Input: dimensioned drawing with shaded views. Units: mm. Origin: part minimum x, y, z. A direction names the side the tool comes from. Coordinates: 2 decimals unless noted, no trailing zeros. Loops run counter-clockwise (first coordinate to the right, second up) from the corner with the lowest first, then second, coordinate; pieces in that order, holes last. Notation, with made-up numbers: M 85.5,-13.5 L 133.5,-13.5 A36 cw 133.5,23.5 Z; hole C -10.5,44.5 d11. An arc over 180 degrees is marked long. Write item = value, one per line. Start each with the question number.
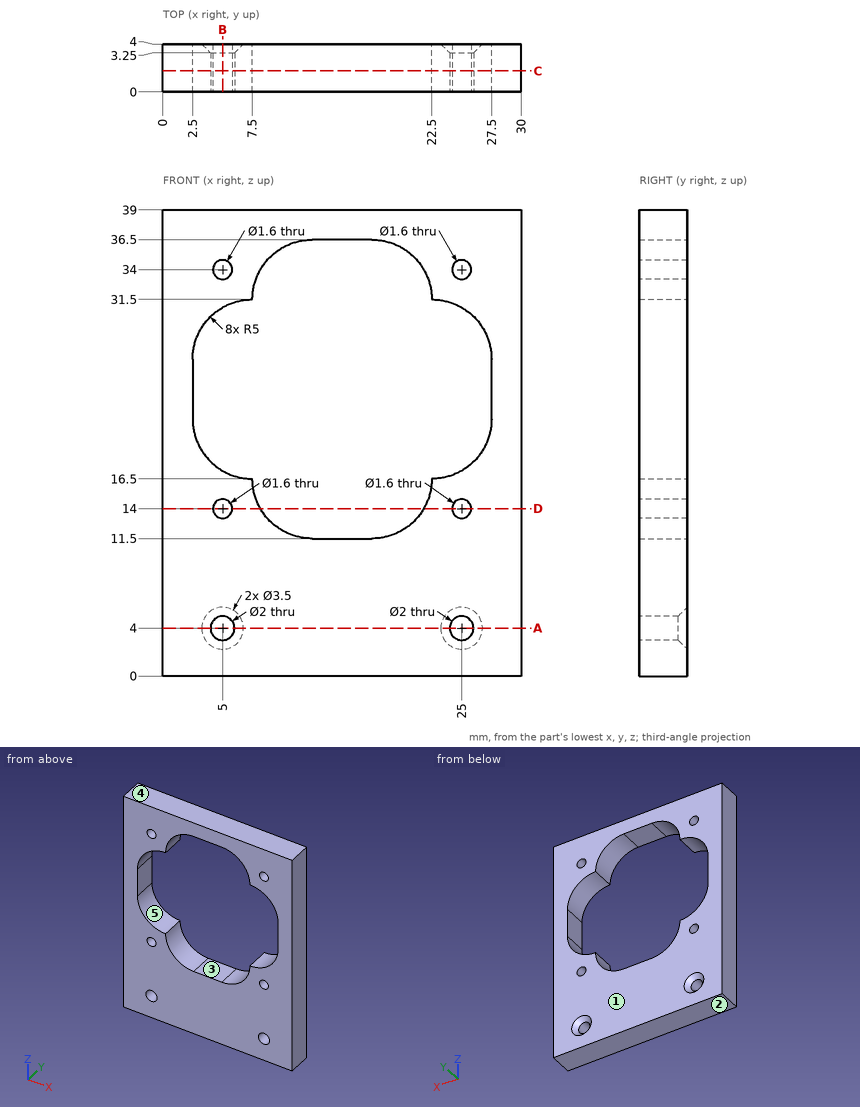
Item 1: Line query: line 1 (Z direction, x = 15.5, y = 1.6); line 2 (X direction, y = 2.85, z = 34); line 3 (Z direction, x = 25, y = 0.9). Output: solid intervals per line, ascending. Write a range as from..to.
Item 2: Pull-direction query (Z, two-part tool) for the marked faces 1, 2 and 3; classes: released by +Z, released by -Z, zero draft, split by the parting line, or undercut.
Item 3: Reachability of the marked faces 4 and 5 from +Z, -Z, +X, -X, +Y, -Y: full face, straight path, thin tool, end or side. Return the list, or none.
Item 4: Section query D-D (z = 14). Return the cut outline in (x, y).
Item 5: Section query C-C (y = 1.75). Count the separate pieces of the cut face and the enclosed holes in it, plus the area to 3 significant figures.
Item 6: Section query A-A (z = 4). Return the cut outline in (x, y).
Item 7: First-contact query: pin 1 (1.4 mm diameter, centred on x = 5, z = 34, fed in from -Y); pin 2 (2.5 mm diameter, centred on x = 25, z = 4, fed in from +Y). Flat tips, straight axial feed; report the tip coordinate or a pass-through.
Item 8: Section query B-B (x = 5). Return the cut outline in (y, z), plus the area to 3 significant figures.
Verdict:
q1.line_1 = 0..11.5, 36.5..39
q1.line_2 = 0..4.2, 5.8..8.17, 21.83..24.2, 25.8..30
q1.line_3 = 0..3, 5..13.2, 14.8..17.17, 30.83..33.2, 34.8..39
q2.face_1 = zero draft
q2.face_2 = released by -Z
q2.face_3 = undercut
q3.face_4 = +Z, +X, -X, +Y, -Y
q3.face_5 = +Y, -Y
q4.outline = M 0,0 L 4.2,0 L 4.2,4 L 0,4 Z; M 5.8,0 L 8.17,0 L 8.17,4 L 5.8,4 Z; M 21.83,0 L 24.2,0 L 24.2,4 L 21.83,4 Z; M 25.8,0 L 30,0 L 30,4 L 25.8,4 Z
q5.separate_pieces = 1
q5.enclosed_holes = 7
q5.area = 674 mm2
q6.outline = M 0,0 L 4,0 L 4,3.25 L 3.25,4 L 0,4 Z; M 6,0 L 24,0 L 24,3.25 L 23.25,4 L 6.75,4 L 6,3.25 Z; M 26,0 L 30,0 L 30,4 L 26.75,4 L 26,3.25 Z
q7.pin_1 = through
q7.pin_2 = 3.5
q8.outline = M 0,0 L 4,0 L 4,2.25 L 3.25,3 L 0,3 Z; M 0,5 L 3.25,5 L 4,5.75 L 4,13.2 L 0,13.2 Z; M 0,14.8 L 4,14.8 L 4,17.17 L 0,17.17 Z; M 0,30.83 L 4,30.83 L 4,33.2 L 0,33.2 Z; M 0,34.8 L 4,34.8 L 4,39 L 0,39 Z
q8.area = 80.0 mm2
